from build123d import *

# Parameters (mm, degrees)
F0_W     = 95.25
F0_H     = 77.47
F0_W_2   = 38.1
F0_H_2   = 26.67
F1_DEPTH = 38.1
F2_R     = 12.7
F3_R     = 8.89
F5_DEPTH = 32.004
F7_DEPTH = 25.4


with BuildPart() as f1:
    # F0 (on Top) → F1 (new body)
    with BuildSketch(Plane.XY):
        with Locations((0, 17.2681905271)):
            Rectangle(F0_W, F0_H)
        with Locations((0, -1.7818094729)):
            Rectangle(F0_W_2, F0_H_2, mode=Mode.SUBTRACT)
    extrude(amount=F1_DEPTH)

    # F2
    f2_edges = [f1.edges().sort_by_distance(p)[0] for p in [
        (47.625, -21.466809, 19.05),
        (-47.625, -21.466809, 19.05),
    ]]
    fillet(f2_edges, radius=F2_R)

    # F3
    f3_edges = [f1.edges().sort_by_distance(p)[0] for p in [
        (19.05, -15.116809, 19.05),
        (19.05, 11.553191, 19.05),
        (-19.05, 11.553191, 19.05),
        (-19.05, -15.116809, 19.05),
    ]]
    fillet(f3_edges, radius=F3_R)

    # F4 (on face) → F5 (cut)
    with BuildSketch(Plane.XY.offset(38.1)):
        with BuildLine():
            ThreePointArc((-41.656, 56.0031905271), (0, 14.3471905271), (41.656, 56.0031905271))
            Line((41.656, 56.0031905271), (-41.656, 56.0031905271))
        make_face()
    extrude(amount=-F5_DEPTH, mode=Mode.SUBTRACT)

    # F6 (on face) → F7 (cut)
    with BuildSketch(Plane.XY.offset(6.096)):
        with BuildLine():
            ThreePointArc((-36.83, 56.0031905271), (0, 19.1731905271), (36.83, 56.0031905271))
            Line((36.83, 56.0031905271), (-36.83, 56.0031905271))
        make_face()
    extrude(amount=-F7_DEPTH, mode=Mode.SUBTRACT)


solid = f1.part
Design review of the part built by this model. Coordinates are the model's own, in mm. A direction names the side the tool comes from. Give positions to 0.01 mm unless a question says otherwise; leave off trailing zeros. Loops run counter-clockwise (first coordinate to the right, second up) from the corner with the lowest first, then second, coordinate; pieces in that order, holes last. Notation, with made-up numbers: (60, 21) - (110, 21) arc R14 ccw to (110, 47) - close; hole circle Ø5 at (83, 46.25). An arc over 180 degrees is marked (long way). Write item = value, one per line.
1) Take a section at A-A on x = 0. State the section outline as (y, z) points, and give its area (3 significant figures).
Result sheet:
outline = (-21.47, 0) - (-15.12, 0) - (-15.12, 38.1) - (-21.47, 38.1) - close; (11.55, 0) - (19.17, 0) - (19.17, 6.1) - (14.35, 6.1) - (14.35, 38.1) - (11.55, 38.1) - close
area = 378 mm2
2) Tool access review of faces 5 (the face through (-44, 56.003, 15)), 6 (the face through (-19.05, -2, 19)), 7 (the face through (-0.916, 14.357, 22.322)): name each direction out of +Z, -Z, +X, -X, +Y, -Y from which nothing blocks a thin tool from reaching the whole face with its end or side.
Result sheet:
face_5 = +Z, -Z, +X, -X, +Y
face_6 = +Z, -Z
face_7 = +Z, +Y
3) Take a section at D-D on x = 13.5. State the section outline as (y, z) points, and give its area (3 significant figures).
Result sheet:
outline = (-21.47, 0) - (-14.47, 0) - (-14.47, 38.1) - (-21.47, 38.1) - close; (10.9, 0) - (21.74, 0) - (21.74, 6.1) - (16.6, 6.1) - (16.6, 38.1) - (10.9, 38.1) - close
area = 515 mm2
4) Take a section at B-B on z = 3. State the section outline as (x, y) points (3 decimals), and give its area (3 significant figures).
Result sheet:
outline = (-47.625, -8.767) arc R12.7 ccw to (-34.925, -21.467) - (34.925, -21.467) arc R12.7 ccw to (47.625, -8.767) - (47.625, 56.003) - (36.83, 56.003) arc R36.83 cw to (-36.83, 56.003) - (-47.625, 56.003) - close; hole (-19.05, -6.227) arc R8.89 ccw to (-10.16, -15.117) - (10.16, -15.117) arc R8.89 ccw to (19.05, -6.227) - (19.05, 2.663) arc R8.89 ccw to (10.16, 11.553) - (-10.16, 11.553) arc R8.89 ccw to (-19.05, 2.663) - close
area = 4,230 mm2
5) To check wall thickness, follow line 1 (X direction, y = -6, z = 5) (3 decimals); line 2 (X direction, y = 8, z = 23.5) (3 decimals); line 3 (Y direction, x = -12, z = 8). State the ranges of each line that lie inside material, in increasing order.
Result sheet:
line_1 = -47.625 to -19.05, 19.05 to 47.625
line_2 = -47.625 to -17.27, 17.27 to 47.625
line_3 = -21.47 to -14.92, 11.36 to 16.11
6) Clearance check with flat-ended pins moving along their axes: pin 1 Ø3 at (x, z) = (-37.5, 12.5) entering from -Y; pin 2 Ø5 at (y, z) = (-13, 9.5) entering from +X; pin 3 Ø2 at (y, z) = (-10.5, 19.5) entering from -X. State where each tip first meets the part, or that it passes through.
Result sheet:
pin_1 = -21.42
pin_2 = 47.51
pin_3 = -47.6
7) Take a section at C-C on y = 31.5. State the section outline as (x, z) points (3 decimals).
Result sheet:
outline = (-47.625, 0) - (-27.496, 0) - (-27.496, 6.096) - (-33.687, 6.096) - (-33.687, 38.1) - (-47.625, 38.1) - close; (27.496, 0) - (47.625, 0) - (47.625, 38.1) - (33.687, 38.1) - (33.687, 6.096) - (27.496, 6.096) - close
8) Draft analysis for pull direction Y (two halves, no side actions). For faces 1 (the face through (-16.377, 9.018, 19.317)), 2 (the face through (-16.38, -12.58, 19.32)), 3 (the face through (0, 18, 6.096)), 4 (the face through (43, 56.003, 15)), state which applies: +Y half, -Y half, draft (parallel to the pull), parting line (faces both ways), or undercut.
Result sheet:
face_1 = undercut
face_2 = undercut
face_3 = draft
face_4 = +Y half
